Source: CAD feature listing. Evaluate the final solid. Frame: model axes, mm. A direction names the side the tool comes from. Give positions to 0.01 mm unless a question says otherwise; leave off trailing zeros. Loops run counter-clockwise (first coordinate to the right, second up) from the corner with the lowest first, then second, coordinate; pieces in that order, holes last. Notation, with made-up numbers: M 49.25,-9.5 L 53.25,-9.5 A21 cw 53.25,2.5 Z; hole C 21.5,49 d2. An arc over 180 degrees is marked long. Answer in a Markdown table with one row per item.
```python
from build123d import *

# Parameters (mm, degrees)
F1_DEPTH  = 349
F2_W      = 9
F2_H      = 87
F3_DEPTH  = 2
F4_W      = 87
F4_H      = 2
F5_DEPTH  = 9
F6_DEPTH  = 11
F8_DEPTH  = 1067
F9_W      = 9
F9_H      = 87
F10_DEPTH = 2


with BuildPart() as f1:
    # F0 (on Top) → F1 (new body)
    with BuildSketch(Plane.XY):
        Polygon((-20, 0), (0, 0), (0, 2), (-9, 2), (-9, 89), (0, 89), (0, 91), (-20, 91), (-20, 89), (-11, 89), (-11, 2), (-20, 2), align=None)
    extrude(amount=F1_DEPTH)

    # F2 (on face) → F3 (join)
    with BuildSketch(Plane.XY.offset(349)):
        Polygon((-20, 0), (0, 0), (0, 2), (-9, 2), (-9, 89), (0, 89), (0, 91), (-20, 91), (-20, 89), (-11, 89), (-11, 2), (-20, 2), align=None)
        with Locations((-15.5, 45.5)):
            Rectangle(F2_W, F2_H)
        with Locations((-4.5, 45.5)):
            Rectangle(F2_W, F2_H)
    extrude(amount=F3_DEPTH)

    # F4 (on face) → F5 (join, through all)
    with BuildSketch(Plane(origin=(-11, 0, 0), x_dir=(0, -1, 0), z_dir=(-1, 0, 0))):
        with Locations((-45.5, 261)):
            Rectangle(F4_W, F4_H)
    extrude(amount=F5_DEPTH)

    # F4 (on face) → F6 (join, through all)
    with BuildSketch(Plane(origin=(-11, 0, 0), x_dir=(0, -1, 0), z_dir=(-1, 0, 0))):
        with Locations((-45.5, 261)):
            Rectangle(F4_W, F4_H)
    extrude(amount=-F6_DEPTH)

    # F7 (on face) → F8 (join)
    with BuildSketch(Plane.XZ):
        Polygon((0, 351), (-20, 351), (-20, 349), (-11, 349), (-11, 262), (-20, 262), (-20, 260), (0, 260), (0, 262), (-9, 262), (-9, 349), (0, 349), align=None)
    extrude(amount=F8_DEPTH)

    # F9 (on face) → F10 (join)
    with BuildSketch(Plane.XZ.offset(1067)):
        with Locations((-15.5, 305.5)):
            Rectangle(F9_W, F9_H)
        with Locations((-4.5, 305.5)):
            Rectangle(F9_W, F9_H)
    extrude(amount=-F10_DEPTH)


solid = f1.part
```
1) Pin query (flat end, axial travel): pin 1 Ø6 at (x, z) = (-16, 52.5) entering from -Y; pin 2 Ø7 at (x, y) = (-5, 31) entering from -Z. Return the tip coordinate at first contact, or that it passes through.
Reply:
| item | result |
|---|---|
| pin 1 | stops at y = 0 |
| pin 2 | stops at z = 260 |
2) Section B-B, the plane y = -196.5. Return loops of the section in (x, z).
Reply:
| item | result |
|---|---|
| outline | M -20,260 L 0,260 L 0,262 L -9,262 L -9,349 L 0,349 L 0,351 L -20,351 L -20,349 L -11,349 L -11,262 L -20,262 Z |
3) Pull-direction query (Y, two-part tool) for faces 5 (the flat face through (-10, -480, 351)), 6 (the flat face through (-9, 45, 305)), 7 (the flat face through (-10, -1067, 306)); classes: released by +Y, released by -Y, zero draft, split by the parting line, or undercut.
Reply:
| item | result |
|---|---|
| face 5 | zero draft |
| face 6 | undercut |
| face 7 | released by -Y |
4) Section A-A, the plane z = 165.5. Return loops of the section in (x, y).
Reply:
| item | result |
|---|---|
| outline | M -20,0 L 0,0 L 0,2 L -9,2 L -9,89 L 0,89 L 0,91 L -20,91 L -20,89 L -11,89 L -11,2 L -20,2 Z |
5) Material intervals for L1, parallel to Y at x = -3, z = 277; L2, parallel to Y at x = -13.25, z = 129.5; L3, parallel to Z at x = -6.5, y = -706, sorted ascending.
Reply:
| item | result |
|---|---|
| L1 | y = -1067 to -1065, 0 to 2, 89 to 91 |
| L2 | y = 0 to 2, 89 to 91 |
| L3 | z = 260 to 262, 349 to 351 |
6) Section C-C, the plane z = 312.5. Return loops of the section in (x, y).
Reply:
| item | result |
|---|---|
| outline | M -20,-1067 L 0,-1067 L 0,-1065 L -9,-1065 L -9,0 L 0,0 L 0,2 L -9,2 L -9,89 L 0,89 L 0,91 L -20,91 L -20,89 L -11,89 L -11,2 L -20,2 L -20,0 L -11,0 L -11,-1065 L -20,-1065 Z |
7) Set-up query: faces 1 (the flat face through (-10, 0, 128)), 2 (the flat face through (-9, 45, 128)), 3 (the flat face through (-11, 46, 128)), 4 (the flat face through (-9, -525, 305)). Return all of +Z, -Z, +X, -X, +Y, -Y with unobstructed straight access to the full face (end or side cutting, diameter ignored); none if empty.
Reply:
| item | result |
|---|---|
| face 1 | -Z, +X, -X, -Y |
| face 2 | -Z, +X |
| face 3 | -Z, -X |
| face 4 | +X |
